Here's the drawing with two shaded views (mm, measured from the low corner). I have some questions. Give positions to 0.01 mm unless a question says otherwise; leave off trailing zeros. Loops run counter-clockwise (first coordinate to the right, second up) from the corner with the lowest first, then second, coordinate; pieces in that order, holes last. Notation, with made-up numbers: M -30.5,13.25 L 27.5,13.25 A23 cw 27.5,39.25 Z; hole C 50.25,-3.75 d2. An arc over 180 degrees is marked long. Put each result on its own line as item: value. Start each with the question number.
1) If we mould it in two halves opening along Z, with no side actions, what happens to the marked faces 1, 2, 3 and 4? For each: +Z half, -Z half, draft (parallel to the pull), parting line (faces both ways), or undercut.
2) Imagine slicing it at A-A (z = 30). Write out the boundary of the cut face in (x, y), then the cut area to 3 significant figures.
3) Imagine slicing it at B-B (x = 40). Write out the boundary of the cut face in (y, z), then the cut area to 3 significant figures.
4) Please list where these lines run through material, in increasing order: line 1 along Z through (x, y) = (40.5, 1); line 2 along Z through (x, y) = (51, 0.75); line 3 along X through (y, z) = (0.75, 20.5). Write a range as from..to.
5) Imagine slicing it at C-C (y = 6). Write out the boundary of the cut face in (x, z), then the cut area to 3 significant figures.
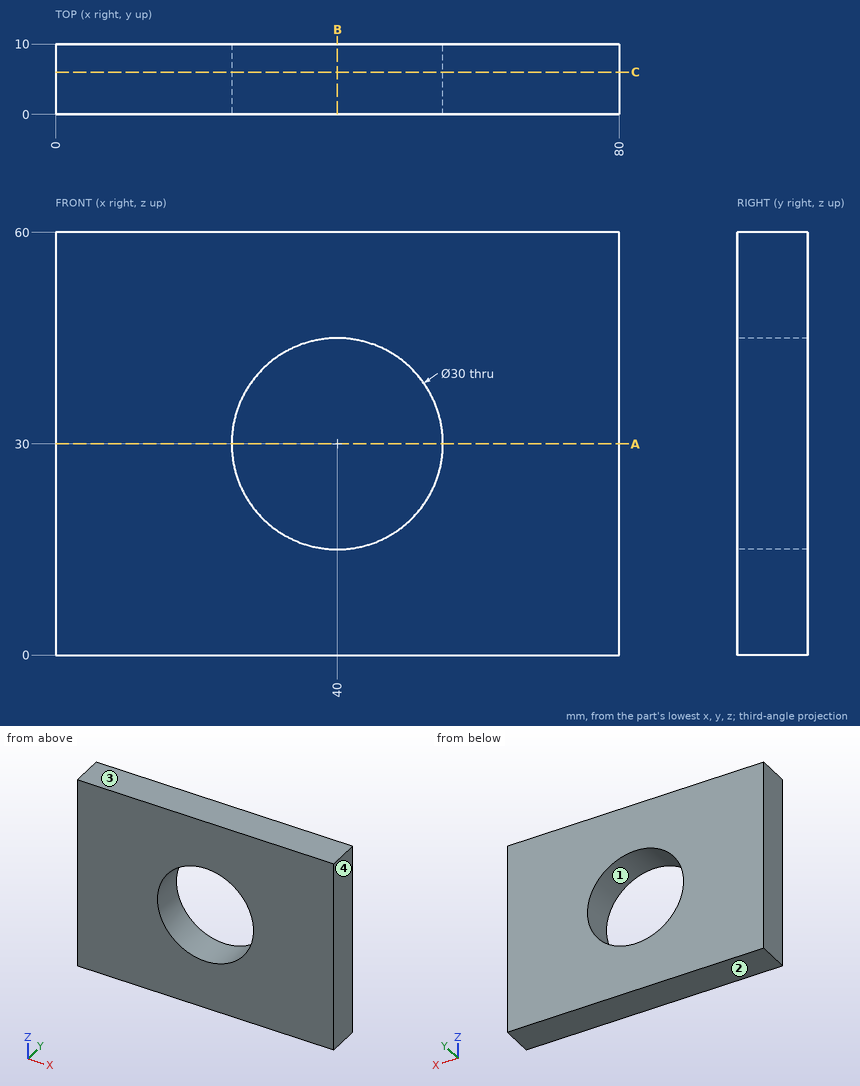
Recorded:
1. face 1: undercut
1. face 2: -Z half
1. face 3: +Z half
1. face 4: draft
2. outline: M 0,0 L 25,0 L 25,10 L 0,10 Z; M 55,0 L 80,0 L 80,10 L 55,10 Z
2. area: 500 mm²
3. outline: M 0,0 L 10,0 L 10,15 L 0,15 Z; M 0,45 L 10,45 L 10,60 L 0,60 Z
3. area: 300 mm²
4. line 1: 0..15.01, 44.99..60
4. line 2: 0..19.8, 40.2..60
4. line 3: 0..28.39, 51.61..80
5. outline: M 0,0 L 80,0 L 80,60 L 0,60 Z; hole C 40,30 d30
5. area: 4,090 mm²
